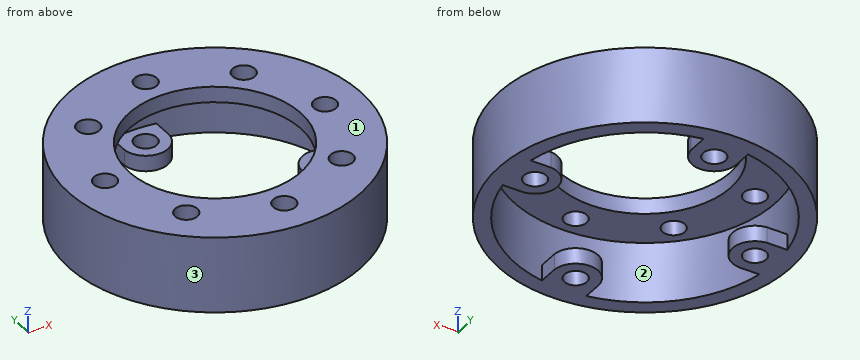
from build123d import *

# Parameters (mm, degrees)
SKETCH2_R           = 5.588
CUT_EXTRUDE1_DEPTH  = 8.874
SKETCH3_R           = 5.588
BOSS_EXTRUDE2_DEPTH = 7.874


with BuildPart() as part:
    # Sketch1 → Revolve1 (revolve)
    with BuildSketch(Plane(origin=(0, 0, 0), x_dir=(1, 0, 0), z_dir=(0, 1, 0))):
        Polygon((73.025, 0), (73.025, 7.874), (73.025, 38.1), (65.278, 38.1), (65.278, 7.874), (42.926, 7.874), (42.926, 0), align=None)
    revolve(axis=Axis((0, 0, -38.1), (0, 0, 1)))

    # Sketch2 → Cut-Extrude1 (cut, through all)
    with BuildSketch(Plane(origin=(0, 0, -7.874), x_dir=(-1, 0, 0), z_dir=(0, 0, -1))):
        with Locations((0, 55.118)):
            Circle(SKETCH2_R)
        with Locations((38.974311565, 38.974311565)):
            Circle(SKETCH2_R)
        with Locations((55.118, 0)):
            Circle(SKETCH2_R)
        with Locations((38.974311565, -38.974311565)):
            Circle(SKETCH2_R)
        with Locations((0, -55.118)):
            Circle(SKETCH2_R)
        with Locations((-38.974311565, -38.974311565)):
            Circle(SKETCH2_R)
        with Locations((-55.118, 0)):
            Circle(SKETCH2_R)
        with Locations((-38.974311565, 38.974311565)):
            Circle(SKETCH2_R)
    extrude(amount=-CUT_EXTRUDE1_DEPTH, mode=Mode.SUBTRACT)

    # Sketch3 → Boss-Extrude2 (add)
    with BuildSketch(Plane(origin=(0, 0, -38.1), x_dir=(-1, 0, 0), z_dir=(0, 0, -1))):
        with BuildLine():
            Line((11.134976442, 54.161299611), (11.134976442, 64.321299611))
            ThreePointArc((11.134976442, 64.321299611), (0, 65.278), (-11.134976442, 64.321299611))
            Line((-11.134976442, 64.321299611), (-11.134976442, 54.161299611))
            ThreePointArc((-11.134976442, 54.161299611), (0, 43.942), (11.134976442, 54.161299611))
        make_face()
        with Locations((0, 55.118)):
            Circle(SKETCH3_R, mode=Mode.SUBTRACT)
        with BuildLine():
            Line((54.161299611, 11.134976442), (64.321299611, 11.134976442))
            ThreePointArc((64.321299611, 11.134976442), (65.278, 0), (64.321299611, -11.134976442))
            Line((64.321299611, -11.134976442), (54.161299611, -11.134976442))
            ThreePointArc((54.161299611, -11.134976442), (43.942, 0), (54.161299611, 11.134976442))
        make_face()
        with Locations((55.118, 0)):
            Circle(SKETCH3_R, mode=Mode.SUBTRACT)
        with BuildLine():
            Line((11.134976442, -54.161299611), (11.134976442, -64.321299611))
            ThreePointArc((11.134976442, -64.321299611), (0, -65.278), (-11.134976442, -64.321299611))
            Line((-11.134976442, -64.321299611), (-11.134976442, -54.161299611))
            ThreePointArc((-11.134976442, -54.161299611), (0, -43.942), (11.134976442, -54.161299611))
        make_face()
        with Locations((0, -55.118)):
            Circle(SKETCH3_R, mode=Mode.SUBTRACT)
        with BuildLine():
            Line((-54.161299611, -11.134976442), (-64.321299611, -11.134976442))
            ThreePointArc((-64.321299611, -11.134976442), (-65.278, 0), (-64.321299611, 11.134976442))
            Line((-64.321299611, 11.134976442), (-54.161299611, 11.134976442))
            ThreePointArc((-54.161299611, 11.134976442), (-43.942, 0), (-54.161299611, -11.134976442))
        make_face()
        with Locations((-55.118, 0)):
            Circle(SKETCH3_R, mode=Mode.SUBTRACT)
    extrude(amount=-BOSS_EXTRUDE2_DEPTH)


solid = part.part
The model under review builds one solid part; all positions refer to its coordinate system, in mm. Face numbers are marked on the shaded views. Round coordinates to 2 decimals unless told otherwise and drop trailing zeros. Loops run counter-clockwise (first coordinate to the right, second up) from the corner with the lowest first, then second, coordinate; pieces in that order, holes last. Notation, with made-up numbers: (30.25, 16.5) -> (55.25, 16.5) arc R22 cw to (55.25, 33.5) -> close; hole circle Ø2 at (24, 53.5). An arc over 180 degrees is marked (long way). Answer as CSV lines item,"result".
1) Add section A-A on y = 0. State how many separate pieces and enclosed holes the cut face has, plus the area to 3 significant figures.
Geometry results:
separate pieces,"6"
enclosed holes,"0"
area,"926 mm²"
2) Draft analysis for pull direction Y (two halves, no side actions). For the marked faces 1, 2 and 3, state which applies: pulls with the +Y half, pulls with the -Y half, needs draft (parallel to the pull), parting line crosses it, or undercut.
Geometry results:
face 1,"needs draft"
face 2,"undercut"
face 3,"parting line crosses it"
3) Add section C-C on x = -21. Write out the cut boundary in (y, z).
Geometry results:
outline,"(-69.94, -38.1) -> (-61.81, -38.1) -> (-61.81, -7.87) -> (-37.44, -7.87) -> (-37.44, 0) -> (-69.94, 0) -> close; (37.44, -7.87) -> (61.81, -7.87) -> (61.81, -38.1) -> (69.94, -38.1) -> (69.94, 0) -> (37.44, 0) -> close"
4) To check wall thickness, follow line 1 along Y through (x, z) = (0, -5) (3 decimals); line 2 along Y through (x, z) = (-0.5, -3); line 3 along X through (y, z) = (-45.5, -36). State the ranges of each line that lie inside material, in increasing order. Write a range as from..to.
Geometry results:
line 1,"y = -73.025..-60.706, -49.53..-42.926, 42.926..49.53, 60.706..73.025"
line 2,"y = -73.02..-60.68, -49.55..-42.92, 42.92..49.55, 60.68..73.02"
line 3,"x = -57.12..-46.81, -5.69..5.69, 46.81..57.12"
5) Add section D-D on y = 26. Write out the cut boundary in (x, z).
Geometry results:
outline,"(-68.24, -38.1) -> (-59.88, -38.1) -> (-59.88, -7.87) -> (-34.16, -7.87) -> (-34.16, 0) -> (-68.24, 0) -> close; (34.16, -7.87) -> (59.88, -7.87) -> (59.88, -38.1) -> (68.24, -38.1) -> (68.24, 0) -> (34.16, 0) -> close"
6) For P1, Ø2, axis at x = -3.5, z = -17, coming from the +Y side; P2, Ø6.5, axis at y = -57, z = -35.5, coming from the +X side; P3, Ø5, axis at y = -17.5, z = -21, coming from the -X side, all flat-tipped, find the tip position at first contact; note any pin that passes through.
Geometry results:
P1,"stops at y = 72.98"
P2,"stops at x = 49.43"
P3,"stops at x = -71.47"
